```python
from build123d import *

# Parameters (mm, degrees)
SKETCH_1_W          = 12
SKETCH_1_H          = 12
SKETCH_1_W_2        = 10
SKETCH_1_H_2        = 10
EXTRUDE_1_DEPTH     = 150
SKETCH_3_R          = 1.55
CUT_EXTRUDE_1_DEPTH = 151.956947505


with BuildPart() as part:
    # 草图1 → 凸台-拉伸1 (new body)
    with BuildSketch(Plane.XY):
        with Locations((6, 6)):
            Rectangle(SKETCH_1_W, SKETCH_1_H)
        with Locations((6, 6)):
            Rectangle(SKETCH_1_W_2, SKETCH_1_H_2, mode=Mode.SUBTRACT)
    extrude(amount=EXTRUDE_1_DEPTH)

    # 草图3 → 切除-拉伸1 (cut, through all)
    with BuildSketch(Plane.YZ.offset(12)):
        with Locations(Location((6, 30, 0), (0, 0, 270))):
            Circle(SKETCH_3_R)
        with Locations(Location((6, 45, 0), (0, 0, 270))):
            Circle(SKETCH_3_R)
        with Locations(Location((6, 60, 0), (0, 0, 270))):
            Circle(SKETCH_3_R)
    extrude(amount=-CUT_EXTRUDE_1_DEPTH, mode=Mode.SUBTRACT)


solid = part.part
```
Source: CAD feature listing. Evaluate the final solid. Frame: model axes, mm. A direction names the side the tool comes from. Coordinates: 2 decimals unless noted, no trailing zeros. Write each loop counter-clockwise with the first axis right and the second up, starting at its lowest first coordinate (ties: lowest second). Pieces come first, ordered by that corner, then holes. Notation, with made-up numbers: (-1, 12.5) - (26, 12.5) arc R30 ccw to (26, 37.5) - close; hole circle Ø11 at (41.25, 1.5). An arc over 180 degrees is marked (long way). Answer as a JSON object with one key per item and string values.
Q1. Section query A-A, the plane x = 7.25. Output: boundary loops of the cut face in (y, z).
Ans:
{"outline": "(0, 0) - (1, 0) - (1, 150) - (0, 150) - close; (11, 0) - (12, 0) - (12, 150) - (11, 150) - close"}
Q2. Section query B-B, the plane z = 128. Output: boundary loops of the cut face in (x, y).
Ans:
{"outline": "(0, 0) - (12, 0) - (12, 12) - (0, 12) - close; hole (1, 1) - (11, 1) - (11, 11) - (1, 11) - close"}
Q3. Set-up query: faces 4 (the cylindrical face through (11.507, 5.406, 28.568)), 5 (the flat face through (6, 1, 74)). Return all of +Z, -Z, +X, -X, +Y, -Y with unobstructed straight access to the full face (end or side cutting, diameter ignored); none if empty.
Ans:
{"face 4": "+X, -X", "face 5": "+Z, -Z"}
Q4. Material intervals for line 1 (Y direction, x = 2.25, z = 141); line 2 (Y direction, x = 11.2, z = 60), sorted ascending. Write a range as [from, to].
Ans:
{"line 1": "y = [0, 1], [11, 12]", "line 2": "y = [0, 4.45], [7.55, 12]"}
Q5. Section query C-C, the plane y = 6. State how many separate pieces and enclosed holes the cut face has, plus the area to 3 significant figures.
Ans:
{"separate pieces": "8", "enclosed holes": "0", "area": "281 mm2"}
Q6. Section query D-D, the plane z = 30. Output: boundary loops of the cut face in (x, y), plus the area to 3 significant figures.
Ans:
{"outline": "(0, 0) - (12, 0) - (12, 4.45) - (11, 4.45) - (11, 1) - (1, 1) - (1, 4.45) - (0, 4.45) - close; (0, 7.55) - (1, 7.55) - (1, 11) - (11, 11) - (11, 7.55) - (12, 7.55) - (12, 12) - (0, 12) - close", "area": "37.8 mm2"}
Q7. Draft query along Y for faces 1 (the flat face through (6, 11, 74)), 2 (the flat face through (6, 12, 74)), 3 (the flat face through (11.2, 6.1, 0)). Return one class per face: released by +Y, released by -Y, zero draft, split by the parting line, or undercut.
Ans:
{"face 1": "undercut", "face 2": "released by +Y", "face 3": "zero draft"}
